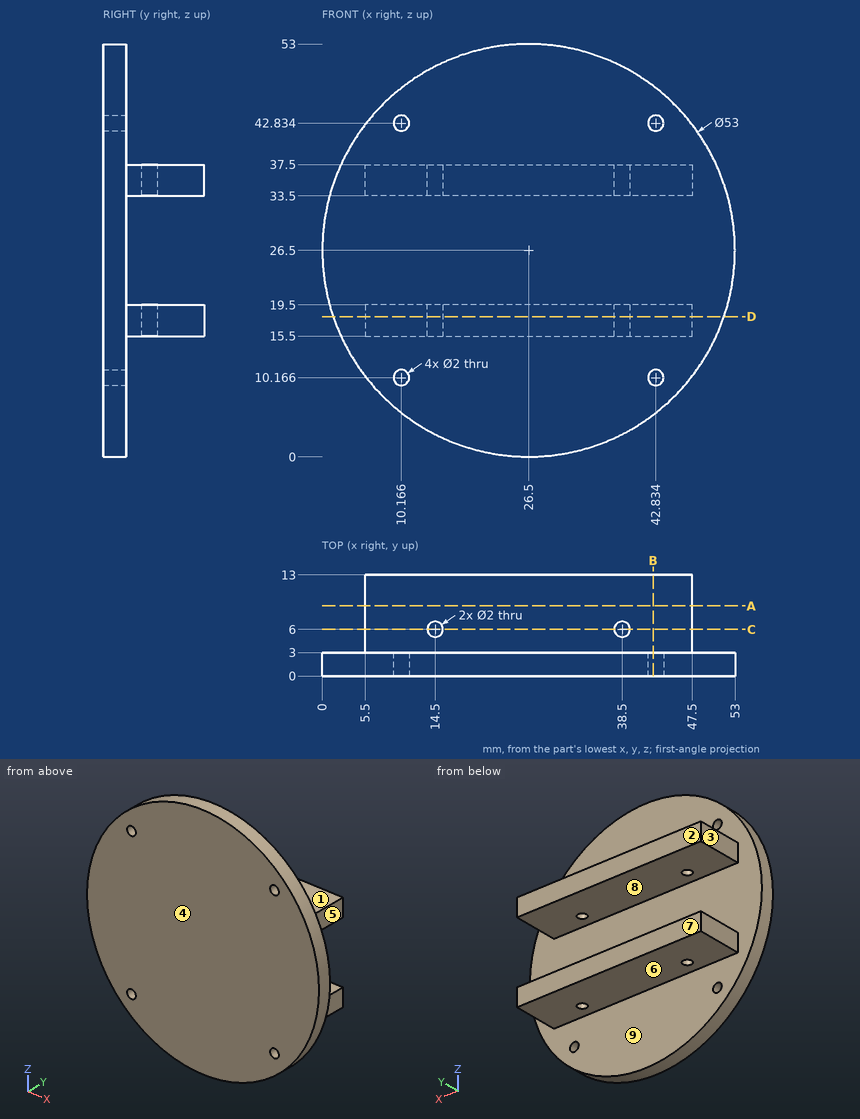
Design review of the part shown in the three views and the two pictorial views. Dimensions are in mm from the part's minimum x, y and z. A direction names the side the tool comes from. Round coordinates to 2 decimals unless told otherwise and drop trailing zeros. Loops run counter-clockwise (first coordinate to the right, second up) from the corner with the lowest first, then second, coordinate; pieces in that order, holes last. Notation, with made-up numbers: (1.5, -24.5) - (14.5, -24.5) arc R11 ccw to (14.5, -11.5) - close; hole circle Ø10 at (-25, -25). An arc over 180 degrees is marked (long way). Use one line per item in the form item = value.
1) We need section A-A on y = 9. Write out the cut boundary in (x, z), then the cut area to 3 significant figures.
Solutions:
outline = (5.5, 15.5) - (47.5, 15.5) - (47.5, 19.5) - (5.5, 19.5) - close; (5.5, 33.5) - (47.5, 33.5) - (47.5, 37.5) - (5.5, 37.5) - close
area = 336 mm2
2) Mouldability with a two-part tool opening along Z and no side actions: class the marked faces 6, 7, 8 and 9 as pulls with the +Z half, pulls with the -Z half, needs draft (parallel to the pull), parting line crosses it, or undercut.
Solutions:
face_6 = pulls with the -Z half
face_7 = needs draft
face_8 = undercut
face_9 = undercut
3) We need section B-B on x = 42.5. Write out the cut boundary in (y, z), then the cut area to 3 significant figures.
Solutions:
outline = (0, 5.38) - (3, 5.38) - (3, 9.22) - (0, 9.22) - close; (0, 11.11) - (3, 11.11) - (3, 15.5) - (13, 15.5) - (13, 19.5) - (3, 19.5) - (3, 33.5) - (13, 33.5) - (13, 37.5) - (3, 37.5) - (3, 41.89) - (0, 41.89) - close; (0, 43.78) - (3, 43.78) - (3, 47.62) - (0, 47.62) - close
area = 195 mm2
4) We need section C-C on y = 6. Write out the cut boundary in (x, z), then the cut area to 3 significant figures.
Solutions:
outline = (5.5, 15.5) - (13.5, 15.5) - (13.5, 19.5) - (5.5, 19.5) - close; (5.5, 33.5) - (13.5, 33.5) - (13.5, 37.5) - (5.5, 37.5) - close; (15.5, 15.5) - (37.5, 15.5) - (37.5, 19.5) - (15.5, 19.5) - close; (15.5, 33.5) - (37.5, 33.5) - (37.5, 37.5) - (15.5, 37.5) - close; (39.5, 15.5) - (47.5, 15.5) - (47.5, 19.5) - (39.5, 19.5) - close; (39.5, 33.5) - (47.5, 33.5) - (47.5, 37.5) - (39.5, 37.5) - close
area = 304 mm2
5) We need section D-D on z = 18. Write out the cut boundary in (x, y), then the cut area to 3 significant figures.
Solutions:
outline = (1.4, 0) - (51.6, 0) - (51.6, 3) - (47.5, 3) - (47.5, 13) - (5.5, 13) - (5.5, 3) - (1.4, 3) - close; hole circle Ø2 at (14.5, 6); hole circle Ø2 at (38.5, 6)
area = 564 mm2
6) Clearance check with flat-ended pins moving along their axes: P1, Ø6, axis at x = 35, z = 11, coming from the +Y side; P2, Ø1.2, axis at y = 7.5, z = 36.5, coming from the -X side; P3, Ø3, axis at x = 14.5, y = 6, coming from the +Z side. State where each tip first meets the part, or that it passes through.
Solutions:
P1 = 3
P2 = 5.5
P3 = 37.5
7) Tool access review of the marked faces 1, 2, 3, 4 and 5: name each direction out of +Z, -Z, +X, -X, +Y, -Y from which nothing blocks a thin tool from reaching the whole face with its end or side.
Solutions:
face_1 = +Z, +X, -X, +Y
face_2 = +Z, -Z, +X, -X, +Y
face_3 = +Z, -Z, -X, +Y
face_4 = +Z, -Z, +X, -X, -Y
face_5 = +Z, -Z, +X, +Y
8) Wall thickness on probe 1 along Y at (x, z) = (38.5, 34.8); probe 2 along Z at (x, y) = (24, 4.25); probe 3 along Y at (x, z) = (21, 21): over which ranges is each line inside the solid? List them lowest first.
Solutions:
probe_1 = 0 to 5, 7 to 13
probe_2 = 15.5 to 19.5, 33.5 to 37.5
probe_3 = 0 to 3
